Model file for the job. Use its own axes, mm. A direction names the side the tool comes from. Round coordinates to 2 decimals unless told otherwise and drop trailing zeros. Order: outer loops, then holes, each group sorted by start corner. A loop starts at its lowest first (then second) coordinate and runs counter-clockwise, first axis right, second up. Notation, with made-up numbers: (88, 29.5) - (96, 29.5) arc R21 cw to (96, 41.5) - close; hole circle Ø7 at (-33, 4). An arc over 180 degrees is marked (long way). Write item = value, one per line. Start each with the question number.
Autodesk Inventor part; units mm, degrees
ref_plane "Start plane" through (0, 0, 30) normal (0, 0, 1) x (1, 0, 0)
ref_plane "End plane" through (0, 0, 611) normal (0, 0, 1) x (1, 0, 0)
ref_plane "Work Plane5" through (340.8, 45, 30) normal (0, 0, -1) x (-1, 0, 0)
ref_plane "Start plane" through (0, 0, 30) normal (0, 0, 1) x (1, 0, 0)
ref_plane "End plane" through (0, 0, 611) normal (0, 0, 1) x (1, 0, 0)
sketch "Sketch" plane through (0, 0, 0) normal (0, 0, 1) x (1, 0, 0)
  line L0 (-20, -13.4) -> (-20, 13.4)
  line L1 (-13.4, 20) -> (13.4, 20)
  line L2 (20, 13.4) -> (20, -13.4)
  line L3 (13.4, -20) -> (-13.4, -20)
  arc A0 (-20, -13.4) -> (-13.4, -20) centre (-13.4, -13.4) ccw
  arc A1 (-13.4, 20) -> (-20, 13.4) centre (-13.4, 13.4) ccw
  arc A2 (20, 13.4) -> (13.4, 20) centre (13.4, 13.4) ccw
  arc A3 (13.4, -20) -> (20, -13.4) centre (13.4, -13.4) ccw
  arc A4 (-13.4, 17) -> (-17, 13.4) centre (-13.4, 13.4) ccw
  line L4 (-13.4, 17) -> (13.4, 17)
  arc A5 (17, 13.4) -> (13.4, 17) centre (13.4, 13.4) ccw
  line L5 (17, 13.4) -> (17, -13.4)
  arc A6 (13.4, -17) -> (17, -13.4) centre (13.4, -13.4) ccw
  line L6 (13.4, -17) -> (-13.4, -17)
  arc A7 (-17, -13.4) -> (-13.4, -17) centre (-13.4, -13.4) ccw
  line L7 (-17, -13.4) -> (-17, 13.4)
  line L8 (0, 22.0873) -> (0, -22.0873) construction
  line L9 (-22.0873, 0) -> (22.0873, 0) construction
  dimension "d7" = 6.6
  dimension "d10" = 40
  dimension "d11" = 40
  dimension "d12" = 3
  dimension "d15" = 20
  dimension "d16" = 20
extrude "Body" add sketch "Sketch" along normal up to surface (581 mm away) from surface at 30
sketch "Sketch3" plane through (0, 0, 0) normal (0, 0, 1) x (1, 0, 0)
  line L0 (0, 0) -> (10, 0)
ref_plane "Work Plane3" through (0, 0, 0) normal (0, -1, 0) x (1, 0, 0)
sketch "Sketch4" plane through (0, 0, 0) normal (0, -1, 0) x (1, 0, 0)
  line L0 (-2, 30) -> (12, 30)
  line L1 (-2, 611) -> (12, 611)
  dimension "d18" = 581
ref_plane "Work Plane5" through (340.8, 45, 30) normal (0, 0, -1) x (-1, 0, 0)
split "Split2" plane through (340.8, 45, 30) removes the side toward (0, 0, -1)
ref_plane "Work Plane6" through (385, -18.4, 611) normal (0, 0, 1) x (1, 0, 0)
split "Split3" plane through (385, -18.4, 611) removes the side toward (0, 0, 1)
equation "\"d7\" = G_IR"
equation "\"d10\" = G_H"
equation "\"d11\" = G_W"
equation "\"d12\" = G_T"
equation "\"d15\" = 0.5 * d10"
equation "\"d16\" = 0.5 * d11"
equation "\"d3\" = G_L"
equation "\"G_W\" = 40"
equation "\"G_H\" = 40"
equation "\"G_T\" = 3"
equation "\"G_IR\" = 6.6"
equation "\"G_L\" = d18"
equation "\"d14\" = G_OFFSET_END + B_L"
equation "\"B_L\" = 651"
properties part number "DIN EN 10305-5 - 40 x 40 x 3  - 581" material "Steel, Mild"
Item 1: Saw through at A-A, the plane x = -7. Give the cut face in (y, z), then the cut area to 3 significant figures.
Item 2: Probe L1, parallel to X at y = 2, z = 304; L2, parallel to Y at x = -15, z = 480. List the from-to ranges inside material, lowest first.
Item 3: Saw through at C-C, the plane z = 467.5. Give the cut face in (x, y).
Item 4: Mould opens along Y. For faces 1 (the face through (0, 20, 316)), 2 (the face through (0, -17, 316)), 3 (the face through (-18, 0, 611)) say: +Y half, -Y half, draft (parallel to the pull), parting line (faces both ways), or undercut.
Item 5: Which spindle directions (+Z, -Z, +X, -X, +Y, -Y) get a long thin tool onto all of the face, cutting with end or side? Do faces 4 (the face through (-17, 0, 316)), 5 (the face through (-20, 0, 316)). Say none if no direction does.
Item 6: Drop a flat-ended pin along its axis: pin 1 (12 mm diameter, centred on x = -0.5, y = 8.5, fed in from +Z). Give the stop position or say it passes through.
Check sheet entries:
q1.outline = (-20, 30) - (-17, 30) - (-17, 611) - (-20, 611) - close; (17, 30) - (20, 30) - (20, 611) - (17, 611) - close
q1.area = 3,490 mm2
q2.L1 = -20 to -17, 17 to 20
q2.L2 = -19.8 to -16.62, 16.62 to 19.8
q3.outline = (-20, -13.4) arc R6.6 ccw to (-13.4, -20) - (13.4, -20) arc R6.6 ccw to (20, -13.4) - (20, 13.4) arc R6.6 ccw to (13.4, 20) - (-13.4, 20) arc R6.6 ccw to (-20, 13.4) - close; hole (-17, -13.4) arc R3.6 ccw to (-13.4, -17) - (13.4, -17) arc R3.6 ccw to (17, -13.4) - (17, 13.4) arc R3.6 ccw to (13.4, 17) - (-13.4, 17) arc R3.6 ccw to (-17, 13.4) - close
q4.face_1 = +Y half
q4.face_2 = undercut
q4.face_3 = draft
q5.face_4 = +Z, -Z
q5.face_5 = +Z, -Z, -X, +Y, -Y
q6.pin_1 = through
